Read the model definition and answer for the solid it produces. Units are mm, in the model's axes. A direction names the side the tool comes from. Coordinates: 2 decimals unless noted, no trailing zeros. Order: outer loops, then holes, each group sorted by start corner. A loop starts at its lowest first (then second) coordinate and runs counter-clockwise, first axis right, second up. Notation, with made-up numbers: (16.25, 53) -> (55.25, 53) arc R25 cw to (55.25, 78) -> close; hole circle Ø6 at (64, 37.25). An arc over 180 degrees is marked (long way). Answer in a Markdown table with one row per item.
from build123d import *

# Parameters (mm, degrees)
F0_R     = 4
F1_DEPTH = 1.5
F2_R     = 0.55
F3_DEPTH = 0.75
F4_R     = 1.05
F5_DEPTH = 25


with BuildPart() as f1:
    # F0 (on Top) → F1 (new body)
    with BuildSketch(Plane.XY):
        Circle(F0_R)
    extrude(amount=F1_DEPTH)

    # F2 (on face) → F3 (cut)
    with BuildSketch(Plane.XY.offset(1.5)):
        with BuildLine():
            ThreePointArc((0, 1.95), (0.388909, 2.111091), (0.55, 2.5))
            ThreePointArc((0.55, 2.5), (-0.388909, 2.888909), (0, 1.95))
        make_face()
        with Locations((-2.165064, 1.25)):
            Circle(F2_R)
        with Locations((-2.165064, -1.25)):
            Circle(F2_R)
        with Locations((2.165064, 1.25)):
            Circle(F2_R)
        with Locations((2.165064, -1.25)):
            Circle(F2_R)
        with Locations((0, -2.5)):
            Circle(F2_R)
    extrude(amount=-F3_DEPTH, mode=Mode.SUBTRACT)

    # F4 (on face) → F5 (cut)
    with BuildSketch(Plane.XY.offset(1.5)):
        Circle(F4_R)
    extrude(amount=-F5_DEPTH, mode=Mode.SUBTRACT)


solid = f1.part
Q1. Given pin 1 (1.4 mm diameter, centred on x = 0, y = 2.5, fed in from +Z); pin 2 (0.9 mm diameter, centred on x = 0, y = 2.5, fed in from +Z), each flat-ended and moving along its own axis, determine where each tip first touches the part or whether it passes through.
Outcome:
| item | result |
|---|---|
| pin 1 | z = 1.5 |
| pin 2 | z = 0.75 |
Q2. The part is cut by section D-D (x = -0.25). Write down the section's boundary in (y, z).
Outcome:
| item | result |
|---|---|
| outline | (-3.99, 0) -> (-1.02, 0) -> (-1.02, 1.5) -> (-2.01, 1.5) -> (-2.01, 0.75) -> (-2.99, 0.75) -> (-2.99, 1.5) -> (-3.99, 1.5) -> close; (1.02, 0) -> (3.99, 0) -> (3.99, 1.5) -> (2.99, 1.5) -> (2.99, 0.75) -> (2.01, 0.75) -> (2.01, 1.5) -> (1.02, 1.5) -> close |
Q3. For a pull along Y with two mould halves and no side action, classify faces 1 (the face through (-0.867, -3.905, 0.74)), 2 (the face through (2, -1, 0.75)), 3 (the face through (1, -1, 1.5)) as pulls with the +Y half, pulls with the -Y half, needs draft (parallel to the pull), parting line crosses it, or undercut.
Outcome:
| item | result |
|---|---|
| face 1 | parting line crosses it |
| face 2 | undercut |
| face 3 | needs draft |
Q4. Consider line 1 (Y direction, x = 0, z = 1.15); line 2 (X direction, y = 2.25, z = 1); line 3 (X direction, y = 0.5, z = 0.7). Determine where each line is inside the solid, lowest interval first.
Outcome:
| item | result |
|---|---|
| line 1 | -4 to -3.05, -1.95 to -1.05, 1.05 to 1.95, 3.05 to 4 |
| line 2 | -3.31 to -0.49, 0.49 to 3.31 |
| line 3 | -3.97 to -0.92, 0.92 to 3.97 |
Q5. The part is cut by section C-C (x = 1.75). Write down the section's boundary in (y, z), then the cut area to 3 significant figures.
Outcome:
| item | result |
|---|---|
| outline | (-3.6, 0) -> (3.6, 0) -> (3.6, 1.5) -> (1.61, 1.5) -> (1.61, 0.75) -> (0.89, 0.75) -> (0.89, 1.5) -> (-0.89, 1.5) -> (-0.89, 0.75) -> (-1.61, 0.75) -> (-1.61, 1.5) -> (-3.6, 1.5) -> close |
| area | 9.71 mm² |
Q6. The part is cut by section A-A (y = 0). Write down the section's boundary in (x, z), then the cut area to 3 significant figures.
Outcome:
| item | result |
|---|---|
| outline | (-4, 0) -> (-1.05, 0) -> (-1.05, 1.5) -> (-4, 1.5) -> close; (1.05, 0) -> (4, 0) -> (4, 1.5) -> (1.05, 1.5) -> close |
| area | 8.85 mm² |
Q7. The part is cut by section B-B (z = 1). Write down the section's boundary in (x, y), then the cut area to 3 significant figures.
Outcome:
| item | result |
|---|---|
| outline | circle Ø8 at (0, 0); hole circle Ø1.1 at (-2.17, -1.25); hole circle Ø1.1 at (-2.17, 1.25); hole circle Ø2.1 at (0, 0); hole circle Ø1.1 at (0, -2.5); hole (0, 1.95) arc R0.55 ccw to (0.55, 2.5) arc R0.55 ccw (long way) to start; hole circle Ø1.1 at (2.17, -1.25); hole circle Ø1.1 at (2.17, 1.25) |
| area | 41.1 mm² |
Q8. For faces 4 (the face through (0, 2.5, 0.75)), 5 (the face through (1, -1, 0)), determine the directions among +Z, -Z, +X, -X, +Y, -Y from which every point of the face is accessible in a straight line to the end or side of a thin tool.
Outcome:
| item | result |
|---|---|
| face 4 | +Z |
| face 5 | -Z, +X, -X, +Y, -Y |
